Can you work these out from the model? Positions are in its coordinate system, mm. A direction names the side the tool comes from. Coordinates: 2 decimals unless noted, no trailing zeros. Write each loop counter-clockwise with the first axis right and the second up, starting at its lowest first coordinate (ties: lowest second). Pieces come first, ordered by that corner, then holes. Notation, with made-up numbers: (59, 57) -> (104, 57) arc R7 cw to (104, 68) -> close; hole circle Ø11 at (-27, -34.75). An arc over 180 degrees is marked (long way). Use one line per item in the form item = value.
Autodesk Inventor part; units mm, degrees
ref_plane "作業平面1" through (-22, 4, 0) normal (0.1788854, 0.9838699, 0) x (0.7333333, -0.1333333, -0.6666667)
ref_plane "YZ Plane" through (0, 0, 0) normal (1, 0, 0) x (0, 1, 0)
ref_plane "XZ Plane" through (0, 0, 0) normal (0, 1, 0) x (-1, 0, 0)
sketch "スケッチ1" plane through (0, 0, 0) normal (0, 1, 0) x (-1, 0, 0)
  line L0 (22, 0) -> (0, 0)
  line L1 (0, 0) -> (0, -41)
  line L2 (0, -41) -> (22, -41)
  line L3 (22, -41) -> (22, 0)
  dimension "d0" = 41
  dimension "d1" = 22
extrude "押し出し1" add sketch "スケッチ1" along normal blind 4
sketch "スケッチ2" plane through (0, 0, 0) normal (1, 0, 0) x (0, 0, -1)
  line L0 (0, 0) -> (41, 0)
  line L1 (41, 0) -> (41, 4)
  line L2 (0, 4) -> (41, 4)
  line L3 (0, 0) -> (0, 4)
  point P0 (20, 0)
ref_plane "作業平面1" through (-22, 4, 0) normal (0.1788854, 0.9838699, 0) x (0.7333333, -0.1333333, -0.6666667)
sketch "スケッチ3" plane through (-22, 4, 0) normal (0.1788854, 0.9838699, 0) x (0.7333333, -0.1333333, -0.6666667)
  line L0 (27.3333, 30.5596) -> (0, 0)
  line L1 (16.6667, -14.9071) -> (44, 15.6525)
  line L2 (16.6667, -14.9071) -> (44, 15.6525)
  line L3 (0, 0) -> (30, 0)
  line L4 (27.3333, 30.5596) -> (30, 0)
  line L5 (-20, -21.3606) -> (60, -21.3606)
  line L6 (60, -21.3606) -> (60, 40)
  line L7 (60, 40) -> (-20, 40)
  line L8 (-20, 40) -> (-20, -21.3606)
  line L9 (16.6667, -14.9071) -> (19.3333, -11.9257)
  line L10 (19.3333, -11.9257) -> (2.6667, 2.9814)
  line L11 (2.6667, 2.9814) -> (0, 0)
  line L12 (0, 0) -> (16.6667, -14.9071)
  line L13 (44, 15.6525) -> (41.3333, 12.6711)
  line L14 (41.3333, 12.6711) -> (24.6667, 27.5782)
  line L15 (24.6667, 27.5782) -> (27.3333, 30.5596)
  line L16 (27.3333, 30.5596) -> (44, 15.6525)
  point P0 (41.3333, 12.6711)
  point P1 (27.8413, 24.7387)
  point P2 (6, 0)
  dimension "d10" = 4
  dimension "d11" = 4
extrude "押し出し2" cut sketch "スケッチ3" along normal through all contours L14 L1 L4 | L1 L10 L3 | L8 L7 L6 L5
sketch "スケッチ4" plane through (0, 4, 0) normal (0, 1, 0) x (1, 0, 0)
  line L0 (0, 20.672) -> (-17.671, 37)
  line L1 (-22, 41) -> (-22, 0)
  line L2 (-17.4545, 4) -> (0, 19.36)
  line L3 (0, 19.36) -> (0, 20.672)
  line L4 (-22, 5.0983) -> (-11, 14.7783)
  line L5 (-11, 14.7783) -> (-11, 25.2537)
  line L6 (-11, 25.2537) -> (-22, 35.4177)
  line L7 (-22, 0) -> (0, 19.36)
  line L8 (0, 20.672) -> (-22, 41)
  line L9 (0, 4) -> (-17.4545, 4)
  line L10 (-17.671, 37) -> (0, 37)
  line L11 (0, 37) -> (0, 41)
  line L12 (0, 41) -> (-22, 41)
  line L13 (-22, 0) -> (0, 0)
  line L14 (0, 0) -> (0, 4)
  point P0 (-11, 20.016)
  point P1 (0, 20.016)
  dimension "d6" = 11
  dimension "d7" = 3.8274
extrude "押し出し3" cut sketch "スケッチ4" against normal through all contours L6 L5 L4 L1
chamfer "面取り1" distance 3 angle 45 2 edges at (-8.7273, 4, -4) (-8.8355, 4, -37)
chamfer "面取り2" distance 3 angle 45 1 edges at (0, 0, -12)
chamfer "面取り3" distance 3 angle 45 1 edges at (0, 0, -28.5)
sketch "スケッチ5" plane through (0, 0, -41) normal (0, 0, -1) x (-1, 0, 0)
  circle A0 centre (5, 2) radius 0.8
  circle A1 centre (17, 2) radius 0.8
  line L0 (0, 0) -> (0, 4)
  line L1 (22, 0) -> (22, 4)
  point P0 (0, 2)
  dimension "d21" = 1.6
  dimension "d22" = 1.6
  dimension "d23" = 5
  dimension "d24" = 5
extrude "押し出し4" cut sketch "スケッチ5" against normal up to surface surface through (-5.5, 2.5, -38.5) normal (0, 0.7071068, 0.7071068)
sketch "スケッチ7" plane through (-22, 0, 0) normal (0, 0, 1) x (1, 0, 0)
  circle A0 centre (17, 2) radius 0.8
  circle A1 centre (5, 2) radius 0.8
  point P0 (22, 0)
extrude "押し出し5" cut sketch "スケッチ7" against normal up to surface surface through (-14.3, 2.5, -2.5) normal (0, 0.7071068, -0.7071068)
equation "\"d11\" = d10"
equation "\"d24\" = d23"
properties part number "chest_cover"
Q1. Thinking about a two-plate mould opening in Z: for faces 1 (the flat face through (-8, 3, -2)), 2 (the flat face through (0, 2, -20)), 3 (the flat face through (-11, 2, -41)), which applies, released by +Z, released by -Z, zero draft, split by the parting line, or undercut?
Return value:
face_1 = undercut
face_2 = zero draft
face_3 = released by -Z
Q2. Suppose I cut it at A-A (x = -14). Write out the boundary of the cut face in (y, z).
Return value:
outline = (0, -41) -> (4, -41) -> (4, -40) -> (2.55, -38.55) -> (2.55, -33.36) -> (4, -33.61) -> (4, -28.03) -> (0, -28.03) -> close; (0, -12.14) -> (4, -12.14) -> (4, -7.04) -> (2.55, -7.27) -> (2.55, -2.45) -> (4, -1) -> (4, 0) -> (0, 0) -> close
Q3. Suppose I cut it at C-C (x = -5). Write out the boundary of the cut face in (y, z).
Return value:
outline = (0, -41) -> (1.2, -41) -> (1.2, -37.2) -> (1, -37) -> (0.91, -37) -> (0.91, -24.77) -> (4, -25.29) -> (4, -14.96) -> (0.91, -15.45) -> (0.91, -4) -> (1, -4) -> (1.2, -3.8) -> (1.2, 0) -> (0, 0) -> close; (2.8, -41) -> (4, -41) -> (4, -40) -> (2.8, -38.8) -> close; (2.8, -2.2) -> (4, -1) -> (4, 0) -> (2.8, 0) -> close
Q4. Suppose I cut it at D-D (x = -1.75). Write out the boundary of the cut face in (y, z).
Return value:
outline = (0, -41) -> (4, -41) -> (4, -40) -> (1, -37) -> (0, -37) -> close; (0, -21.62) -> (4, -22.29) -> (4, -17.82) -> (0, -18.46) -> close; (0, -4) -> (1, -4) -> (4, -1) -> (4, 0) -> (0, 0) -> close
Q5. If I drill on line 1 (X direction, y = 2, z = -39.8); line 2 (Z direction, x = -3.5, y = 2.9); line 3 (Z direction, x = -7.75, y = 2.4), over which ranges is the centre line in solid material (lowest first)? Write a range as from..to.
Return value:
line_1 = -22..-17.8, -16.2..-5.8, -4.2..0
line_2 = -41..-38.9, -23.72..-16.46, -2.1..0
line_3 = -41..-38.4, -27.56..-12.8, -2.6..0
Q6. Will these pins go through, and if not, where does the flat tip stop? pin 1 (1 mm diameter, centred on x = -17, y = 2, fed in from +Z); pin 2 (4 mm diameter, centred on x = -3, z = -12.5, fed in from +Y); pin 3 (1.8 mm diameter, centred on x = -5, y = 2, fed in from +Z); pin 4 (1.5 mm diameter, centred on y = 1, z = -27, fed in from +X).
Return value:
pin_1 = -2.5
pin_2 = 0.91
pin_3 = 0
pin_4 = -2.95
Q7. For faces 4 (the flat face through (-8.06, 2.66, -12.48)), 5 (the cylindrical face through (-4.83, 1.22, -39.55)), 6 (the flat face through (-16.42, 2.03, -30.26)), which set-ups out of +Z, -Z, +X, -X, +Y, -Y let a thin tool reach every point of the face, with its end or its side?
Return value:
face_4 = +X
face_5 = -Z
face_6 = -X, +Y, -Y
Q8. Suppose I cut it at B-B (y = 2). Give the number of separate pieces and of enclosed holes in the cut face, then the cut area to 3 significant figures.
Return value:
separate_pieces = 3
enclosed_holes = 0
area = 390 mm2
